Build history of the part. All positions in model axes, mm. A direction names the side the tool comes from. Coordinates: 2 decimals unless noted, no trailing zeros. Order: outer loops, then holes, each group sorted by start corner. A loop starts at its lowest first (then second) coordinate and runs counter-clockwise, first axis right, second up. Notation, with made-up numbers: (-21.75, -9.5) - (32.25, -9.5) arc R14 ccw to (32.25, 8.5) - close; hole circle Ø8 at (24, 61). An arc over 180 degrees is marked (long way). Return JSON: item names as keys, results as strings.
Autodesk Inventor part; units mm, degrees
ref_plane "YZ Plane" through (0, 0, 0) normal (1, 0, 0) x (0, 1, 0)
ref_plane "XZ Plane" through (0, 0, 0) normal (0, 1, 0) x (-1, 0, 0)
ref_plane "XY Plane" through (0, 0, 0) normal (0, 0, 1) x (1, 0, 0)
sketch "Skizze1" plane through (0, 0, 0) normal (0, 0, 1) x (1, 0, 0)
  line L0 (10, 0) -> (-48, 0)
  line L1 (-55, 5) -> (0, 5)
  line L2 (0, 5) -> (0, 3)
  line L3 (0, 3) -> (10, 3)
  line L4 (10, 3) -> (10, 0)
  line L5 (-55, 5) -> (-55, 2)
  line L6 (-55, 2) -> (-48, 2)
  line L7 (-48, 2) -> (-48, 0)
  point P0 (0, 0)
  point P1 (0, 4)
  dimension "d0" = 10
  dimension "d2" = 10
  dimension "d3" = 6
  dimension "d8" = 55
  dimension "d9" = 4
  dimension "d12" = 7
revolve "Umdrehung1" add sketch "Skizze1" angle 360 about axis through (10, 0, 0) along (-1, 0, 0)
thread "Gewinde2"
thread "Gewinde3"
properties part number "Bolzen" material "Eisen, Grau"
1. Probe L1, parallel to Y at x = -50, z = 0; L2, parallel to X at y = -3.25, z = -2.5. List the from-to ranges inside material, lowest first.
Check values:
{"L1": "-5 to -2, 2 to 5", "L2": "-55 to 0"}
2. Cut at A-A on z = 0. Give the cut face in (x, y).
Check values:
{"outline": "(-55, -5) - (0, -5) - (0, -3) - (10, -3) - (10, 3) - (0, 3) - (0, 5) - (-55, 5) - (-55, 2) - (-48, 2) - (-48, -2) - (-55, -2) - close"}
3. Cut at C-C on x = -42. Give the cut face in (y, z).
Check values:
{"outline": "circle Ø10 at (0, 0)"}
4. Drop flat-ended pins along their axis: pin 1 (1 mm diameter, centred on x = -14, z = -3, fed in from +Y); pin 2 (1.5 mm diameter, centred on x = -22.5, y = 3, fed in from -Z); pin 3 (1 mm diameter, centred on x = -23, z = 1, fed in from -Y); pin 4 (4.5 mm diameter, centred on y = 0, z = 0, fed in from -X). Give the stop position or say it passes through.
Check values:
{"pin 1": "y = 4.33", "pin 2": "z = -4.47", "pin 3": "y = -4.97", "pin 4": "x = -55"}
5. Tool access for faces 1 (the flat face through (10, 0, 0)), 2 (the cylindrical face through (-51, 0, -2)), 3 (the flat face through (0, 3.3, -0.1)): list every direction of +Z, -Z, +X, -X, +Y, -Y with a clear straight run to the whole face (end or side of a thin tool).
Check values:
{"face 1": "+Z, -Z, +X, +Y, -Y", "face 2": "-X", "face 3": "+X"}
